The listing builds one solid part. Answer for the finished solid, in the listing's coordinates (mm). Face numbers are marked on the shaded views. A direction names the side the tool comes from. Round coordinates to 2 decimals unless told otherwise and drop trailing zeros. Write each loop counter-clockwise with the first axis right and the second up, starting at its lowest first coordinate (ties: lowest second). Pieces come first, ordered by that corner, then holes.
Item 1: A tool of negligible diameter and unlimited length cuts with its end or side. For the marked faces 5 and 6, from which of +Z, -Z, +X, -X, +Y, -Y can it reach the whole face along a straight path? Write none if from no direction.
Item 2: Each of these flat-tipped pins is pushed along its axis until it touches: pin 1 (8 mm diameter, centred on x = 5, z = 11.5, fed in from -Y); pin 2 (1.9 mm diameter, centred on x = 10, z = 0, fed in from +Y); pin 3 (8 mm diameter, centred on y = 0, z = 0, fed in from -X); pin 4 (8 mm diameter, centred on x = 5.5, y = -9, fed in from -Z) (3 decimals). Where does it stop, or does it pass through?
Item 3: Find section B-B on y = -36.5. Give the vertices of the cut face in (x, z) (3 decimals).
Item 4: Find section A-A on x = 10. Give the vertices of the cut face in (y, z) (3 decimals), then the cut area to 3 significant figures.
Item 5: For a pull along X with two mould halves and no side action, classify the marked faces 1, 2, 3 and 4 as +X half, -X half, draft (parallel to the pull), parting line (faces both ways), or undercut.
Item 6: Find the intervals of material crossed by probe 1 along Y at (x, z) = (5.45, 0); probe 2 along Z at (x, y) = (10, -40) (3 decimals); probe 3 along X at (y, z) = (-7.5, -1.5), in increasing order.
Item 7: Find section D-D on x = 14. Give the vertices of the cut face in (y, z), then the cut area to 3 significant figures.
Item 8: Find section C-C on x = 17.25. Give the vertices of the cut face in (y, z).
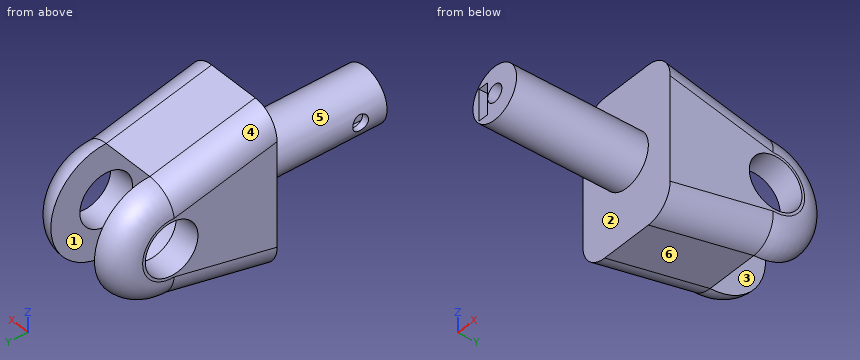
Autodesk Inventor part; units mm, degrees
ref_plane "YZ Plane" through (0, 0, 0) normal (1, 0, 0) x (0, 1, 0)
ref_plane "XZ Plane" through (0, 0, 0) normal (0, 1, 0) x (-1, 0, 0)
ref_plane "XY Plane" through (0, 0, 0) normal (0, 0, 1) x (1, 0, 0)
sketch "Sketch1" plane through (0, 0, 0) normal (1, 0, 0) x (0, 1, 0)
  circle A0 centre (0, 0) radius 5
  circle A1 centre (0, 0) radius 10.5
  line L0 (0, 0) -> (-20, 0)
  line L1 (-20, 0) -> (-20, -15)
  line L2 (-20, -15) -> (-20, 15)
  line L3 (-20, 15) -> (0, 10.5)
  line L4 (0, -10.5) -> (-20, -15)
  dimension "d0" = 10
  dimension "d1" = 21
  dimension "d2" = 20
  dimension "d3" = 15
  dimension "d4" = 30
extrude "Extrusion1" add sketch "Sketch1" along normal blind 5
sketch "Sketch2" plane through (5, 0, 0) normal (1, 0, 0) x (0, 0, -1)
  arc A0 (10.5, 0) -> (-10.5, 0) centre (0, 0) ccw
  circle A1 centre (0, 0) radius 10.5
  line L0 (-10.5, 0) -> (-15, -20)
  line L1 (-10.5, 0) -> (-15, -20)
  line L2 (15, -20) -> (10.5, 0)
  line L3 (-15, -20) -> (15, -20)
  line L4 (15, -20) -> (10.5, 0)
  point P0 (-10.5, 0)
extrude "Extrusion2" add sketch "Sketch2" along normal blind 10 contours L2 L3 L0 A1
sketch "Sketch4" plane through (15, 0, 0) normal (1, 0, 0) x (0, 0, -1)
  circle A0 centre (0, 0) radius 5
  circle A1 centre (0, 0) radius 10.5
  line L0 (15, -20) -> (10.5, 0)
  line L1 (10.5, 0) -> (15, -20)
  line L2 (-15, -20) -> (15, -20)
  line L3 (15, -20) -> (-15, -20)
  line L4 (-10.5, 0) -> (-15, -20)
  line L5 (-15, -20) -> (-10.5, 0)
extrude "Extrusion3" add sketch "Sketch4" along normal blind 5
sketch "Sketch5" plane through (0, -20, -15) normal (0, -1, 0) x (1, 0, 0)
  line L0 (20, 4.5) -> (20, 25.5)
  line L1 (20, 15) -> (0, 15)
  circle A0 centre (10, 15) radius 5
  dimension "d11" = 10
extrude "Extrusion4" add sketch "Sketch5" along normal blind 25
fillet "Fillet1" radius 5 6 edges at (20, -10, 12.75) (20, -10, -12.75) (20, 10.5, 0) (0, 10.5, 0) (0, -10, -12.75) (0, -10, 12.75)
sketch "Sketch6" plane through (10, -45, 0) normal (0, -1, 0) x (1, 0, 0)
  circle A0 centre (0, 0) radius 5
  circle A1 centre (0, 0) radius 1.625
  point P0 (-10, 0)
  dimension "d15" = 3.25
extrude "Extrusion5" cut sketch "Sketch6" against normal blind 20 contours A1
sketch "Sketch7" plane through (0, 0, 0) normal (1, 0, 0) x (0, 1, 0)
  line L0 (-45, 5) -> (-45, -5)
  line L1 (-45, 0) -> (-40, 0)
  circle A0 centre (-40, 0) radius 1.5
  point P0 (0, 0)
  dimension "d18" = 5
  dimension "d19" = 3
extrude "Extrusion6" cut sketch "Sketch7" along normal blind 10
sketch "Sketch8" plane through (10, -45, 0) normal (0, -1, 0) x (1, 0, 0)
  circle A0 centre (0, 0) radius 1.625
  line L0 (-1.625, 0) -> (-1.625, 3)
  line L1 (-1.625, 3) -> (-3.625, 3)
  line L2 (-3.625, 3) -> (-3.625, -3)
  line L3 (-3.625, -3) -> (-1.625, -3)
  line L4 (-1.625, -3) -> (-1.625, 0)
  point P0 (-10, 0)
  dimension "d22" = 3
  dimension "d23" = 2
  dimension "d24" = 6
extrude "Extrusion7" cut sketch "Sketch8" against normal blind 10 contours L4 L3 L2 L1 L0
properties part number "wrist"
Check values:
1. face 5: -Y
1. face 6: -Z, +X, -X, +Y
2. pin 1: stops at y = -20
2. pin 2: stops at y = -10.46
2. pin 3: passes through
2. pin 4: stops at z = -13.425
3. outline: circle Ø10 at (10, 0); hole (6.375, -3) - (8.375, -3) - (8.375, 3) - (6.375, 3) - close; hole circle Ø3.25 at (10, 0)
4. outline: (-45, -5) - (-20, -5) - (-20, -15) - (0, -10.5) arc R10.5 cw to (0, 10.5) - (-20, 15) - (-20, 5) - (-45, 5) - (-45, 1.625) - (-25, 1.625) - (-25, -1.625) - (-45, -1.625) - close
4. area: 522 mm2
5. face 1: undercut
5. face 2: draft
5. face 3: undercut
5. face 4: -X half
6. probe 1: y = -45 to -41.5, -38.5 to -10.5
6. probe 2: z = -5 to -1.625, 1.625 to 5
6. probe 3: x = 0 to 5, 15 to 20
7. outline: (-45, -3) - (-20, -3) - (-20, -15) - (0, -10.5) arc R10.5 cw to (0, 10.5) - (-20, 15) - (-20, 3) - (-45, 3) - close
7. area: 487 mm2
8. outline: (-20, -14.45) - (-0.06, -9.97) arc R9.97 ccw (long way) to (-0.06, 9.97) - (-20, 14.45) - close; hole circle Ø10 at (0, 0)
